Read the model definition and answer for the solid it produces. Units are mm, in the model's axes. Face numbers are marked on the shaded views. A direction names the side the tool comes from. Round coordinates to 2 decimals unless told otherwise and drop trailing zeros. Order: outer loops, then holes, each group sorted by start corner. A loop starts at its lowest first (then second) coordinate and runs counter-clockwise, first axis right, second up. Notation, with made-up numbers: M 70,-27 L 103,-27 A27 ccw 103,-11 Z; hole C -34.5,70 d11. An arc over 180 degrees is marked long. Answer as CSV lines item,"result".
```python
from build123d import *

# Parameters (mm, degrees)
F0_W     = 245
F0_H     = 91
F1_DEPTH = 17.5
F2_W     = 243.4
F2_H     = 89.4
F3_DEPTH = 15.1
F4_W     = 0.8
F4_H     = 89.4
F5_DEPTH = 15.1
F6_W     = 239
F6_H     = 85
F7_DEPTH = 0.2


with BuildPart() as f1:
    # F0 (on Top) → F1 (new body)
    with BuildSketch(Plane.XY):
        Rectangle(F0_W, F0_H)
    extrude(amount=F1_DEPTH)

    # F2 (on face) → F3 (cut)
    with BuildSketch(Plane.XY.offset(17.5)):
        Rectangle(F2_W, F2_H)
    extrude(amount=-F3_DEPTH, mode=Mode.SUBTRACT)

    # F4 (on face) → F5 (join)
    with BuildSketch(Plane.XY.offset(2.4)):
        Rectangle(F4_W, F4_H)
    extrude(amount=F5_DEPTH)

    # F6 (on face) → F7 (cut)
    with BuildSketch(Plane(origin=(0, 0, 0), x_dir=(1, 0, 0), z_dir=(0, 0, -1))):
        Rectangle(F6_W, F6_H)
    extrude(amount=-F7_DEPTH, mode=Mode.SUBTRACT)


solid = f1.part
```
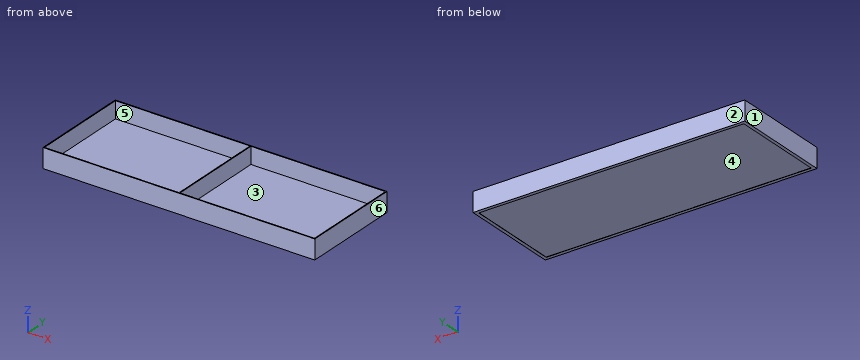
Item 1: A flat-ended cylindrical pin translates along its axis: pin 1 (4 mm diameter, centred on x = 60, y = 28, fed in from -Z). Find the tip coordinate at first contact, or state that the pin passes through.
Ans:
pin 1,"z = 0.2"
Item 2: A cutting plane is placed at B-B, the plane x = 21. Determine the outline of the cut face in (y, z), and give its area (3 significant figures).
Ans:
outline,"M -45.5,0 L -42.5,0 L -42.5,0.2 L 42.5,0.2 L 42.5,0 L 45.5,0 L 45.5,17.5 L 44.7,17.5 L 44.7,2.4 L -44.7,2.4 L -44.7,17.5 L -45.5,17.5 Z"
area,"226 mm2"
Item 3: A tool of negligible diameter and unlimited length cuts with its end or side. For the marked faces 4, 5 and 6, from which of +Z, -Z, +X, -X, +Y, -Y can it reach the whole face along a straight path? Write none if from no direction.
Ans:
face 4,"-Z"
face 5,"+Z"
face 6,"+Z, -Z, +X, +Y, -Y"
Item 4: Determine the mould class of the marked faces 1, 2 and 3 for opening direction Y: +Y half, -Y half, draft (parallel to the pull), parting line (faces both ways), or undercut.
Ans:
face 1,"draft"
face 2,"+Y half"
face 3,"undercut"
Item 5: A cutting plane is placed at A-A, the plane z = 5.5. Determine the outline of the cut face in (x, y).
Ans:
outline,"M -122.5,-45.5 L 122.5,-45.5 L 122.5,45.5 L -122.5,45.5 Z; hole M -121.7,-44.7 L -0.4,-44.7 L -0.4,44.7 L -121.7,44.7 Z; hole M 0.4,-44.7 L 121.7,-44.7 L 121.7,44.7 L 0.4,44.7 Z"
Item 6: Find the intervals of material crossed by probe 1 along X at (y, z) = (40.5, 8.5); probe 2 along Y at (x, z) = (104, 12); probe 3 along Z at (x, y) = (54.5, -14), in increasing order. Write a range as [from, to].
Ans:
probe 1,"[-122.5, -121.7], [-0.4, 0.4], [121.7, 122.5]"
probe 2,"[-45.5, -44.7], [44.7, 45.5]"
probe 3,"[0.2, 2.4]"
Item 7: A cutting plane is placed at C-C, the plane y = 19. Determine the outline of the cut face in (x, z), and give its area (3 significant figures).
Ans:
outline,"M -122.5,0 L -119.5,0 L -119.5,0.2 L 119.5,0.2 L 119.5,0 L 122.5,0 L 122.5,17.5 L 121.7,17.5 L 121.7,2.4 L 0.4,2.4 L 0.4,17.5 L -0.4,17.5 L -0.4,2.4 L -121.7,2.4 L -121.7,17.5 L -122.5,17.5 Z"
area,"576 mm2"
